from build123d import *

# Parameters (mm, degrees)
BOSS_EXTRUDE1_DEPTH        = 19.05
F_8_0_199_DIAMETER_HOLE1_D = 5.0546
SKETCH4_R                  = 1.016
SKETCH4_W                  = 13.589
SKETCH4_H                  = 8.89
CUT_EXTRUDE1_DEPTH         = 24.89121573


with BuildPart() as part:
    # Sketch1 → Boss-Extrude1 (new body)
    with BuildSketch(Plane(origin=(0, 0, 0), x_dir=(0, 0, -1), z_dir=(1, 0, 0))):
        Polygon((-14.980334091, -13.49375), (-14.980334091, 0), (-9.900334091, 0), (-9.900334091, 12.7), (-9.106584091, 12.7), (-9.106584091, -0.79375), (-14.186584091, -0.79375), (-14.186584091, -13.49375), align=None)
    extrude(amount=BOSS_EXTRUDE1_DEPTH)

    # #8 (0.199) Diameter Hole1 (through all)
    with Locations(Plane(origin=(9.525, 6.35, 9.900334091), x_dir=(1, 0, 0), z_dir=(0, 0, 1))):
        with Locations((0, 0)):
            Hole(F_8_0_199_DIAMETER_HOLE1_D / 2)

    # Sketch4 → Cut-Extrude1 (cut, through all)
    with BuildSketch(Plane(origin=(0, 0, 14.186584091), x_dir=(-1, 0, 0), z_dir=(0, 0, -1))):
        with Locations(Location((-15.875, -9.04875, 0), (0, 0, 90))):
            Circle(SKETCH4_R)
        with Locations((-6.7945, -9.04875)):
            Rectangle(SKETCH4_W, SKETCH4_H)
    extrude(amount=-CUT_EXTRUDE1_DEPTH, mode=Mode.SUBTRACT)


solid = part.part
Geometry: final body of the model. Coordinates: model frame, mm. A direction names the side the tool comes from. Give positions to 0.01 mm unless a question says otherwise; leave off trailing zeros. Write each loop counter-clockwise with the first axis right and the second up, starting at its lowest first coordinate (ties: lowest second). Pieces come first, ordered by that corner, then holes.
(1) Mould query, pull axis Y, two halves, no side actions, for faces 4 (the cylindrical face through (16.73, -8.5, 14.58)), 5 (the flat face through (12, -4, 14.187)), 6 (the flat face through (9, 0, 12)). Classes: released by +Y, released by -Y, zero draft, split by the parting line, or undercut.
(2) Cut plane B-B, the plane x = 12.75. Return loops of the section in (y, z), then the cut area to 3 significant figures.
(3) Cut plane A-A, the plane y = 6.35. Return loops of the section in (x, z), then the cut area to 3 significant figures.
(4) Ray query, line 1 (Z direction, x = 10, y = -3.5); line 2 (Y direction, x = 4.5, z = 12); line 3 (Z direction, x = 6, y = 1). Return the intervals inside material, ascending.
(5) Access query for faces 1 (the flat face through (7, 8, 9.9)), 2 (the flat face through (7, 5, 9.107)), 3 (the flat face through (9, -0.794, 12)). Directions: +Z, -Z, +X, -X, +Y, -Y. A direction counts if a zero-diameter tool reaches every point of the face in a straight line with its end or side. Return the directions, or none.
(6) Cut plane C-C, the plane x = 7.75. Return loops of the section in (y, z), then the cut area to 3 significant figures.
(7) Cut plane D-D, the plane y = -2.25. Return loops of the section in (x, z).
(8) First-contact query: P1, Ø3, axis at x = 15, z = 10, coming from the -Y side; P2, Ø1.5, axis at x = 5.5, z = 12.5, coming from the +Y side; P3, Ø10, axis at x = 14, y = 6, coming from the +Z side; P4, Ø1.2, axis at x = 15.88, y = -9.05, coming from the -Z side. Flat tips, straight axial feed; report the tip coordinate or a pass-through.
Values follow:
1. face 4: undercut
1. face 5: zero draft
1. face 6: released by +Y
2. outline: (-4.6, 14.19) - (-0.79, 14.19) - (-0.79, 9.11) - (12.7, 9.11) - (12.7, 9.9) - (0, 9.9) - (0, 14.98) - (-4.6, 14.98) - close
2. area: 17.8 mm2
3. outline: (0, 9.11) - (7, 9.11) - (7, 9.9) - (0, 9.9) - close; (12.05, 9.11) - (19.05, 9.11) - (19.05, 9.9) - (12.05, 9.9) - close
3. area: 11.1 mm2
4. line 1: z = 14.19 to 14.98
4. line 2: y = -0.79 to 0
4. line 3: z = 9.11 to 9.9
5. face 1: +Z, +X, -X, +Y
5. face 2: -Z, +X, -X, +Y, -Y
5. face 3: -Z, +X, -X, -Y
6. outline: (-4.6, 14.19) - (-0.79, 14.19) - (-0.79, 9.11) - (4.55, 9.11) - (4.55, 9.9) - (0, 9.9) - (0, 14.98) - (-4.6, 14.98) - close; (8.15, 9.11) - (12.7, 9.11) - (12.7, 9.9) - (8.15, 9.9) - close
6. area: 14.9 mm2
7. outline: (0, 14.19) - (19.05, 14.19) - (19.05, 14.98) - (0, 14.98) - close
8. P1: stops at y = -0.79
8. P2: stops at y = 0
8. P3: stops at z = 9.9
8. P4: passes through
